Source: three-view drawing plus pictorial views. Frame: mm from the lowest corner of the part. A direction names the side the tool comes from. Coordinates: 2 decimals unless noted, no trailing zeros. Write each loop counter-clockwise with the first axis right and the second up, starting at its lowest first coordinate (ties: lowest second). Pieces come first, ordered by that corner, then holes. Notation, with made-up numbers: M 76.5,37 L 115.5,37 A24 cw 115.5,67 Z; hole C 26,3 d2. An arc over 180 degrees is marked long. Answer as a JSON object with one key per item and string values. Group by question number.
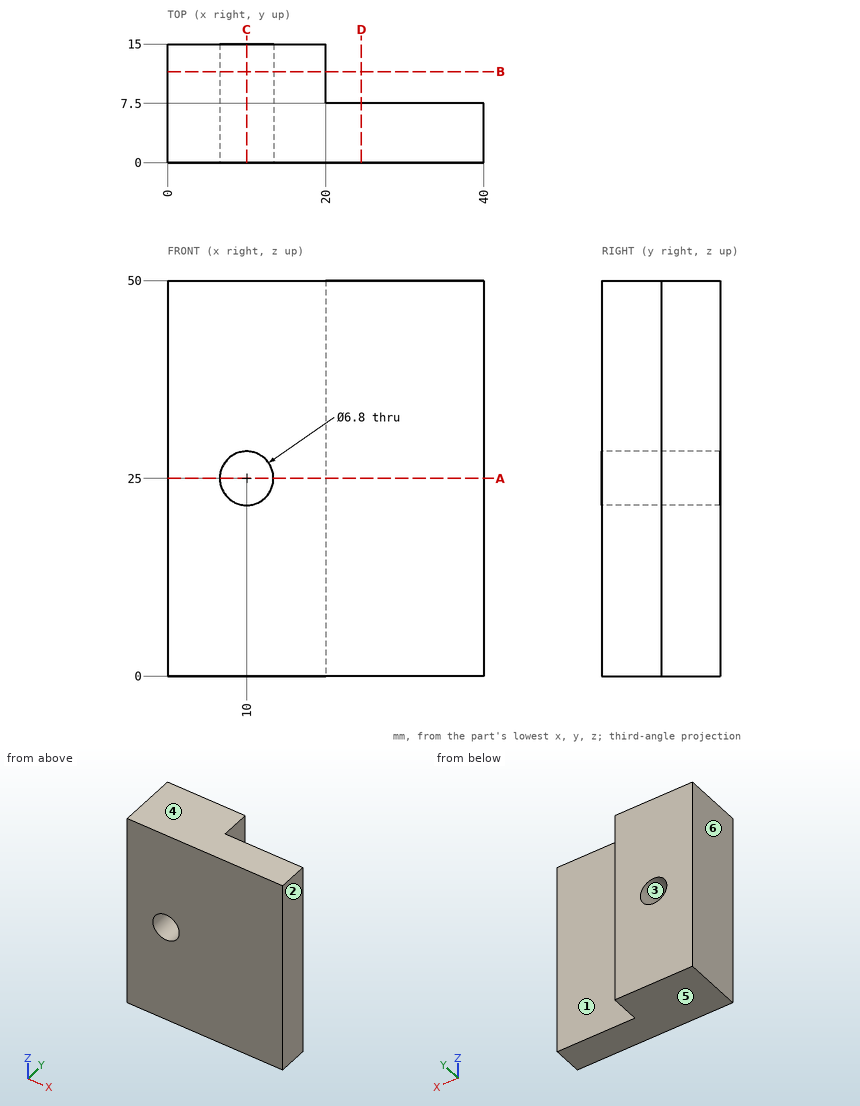
Q1. Pin query (flat end, axial travel): pin 1 Ø2 at (x, y) = (30.5, 2.5) entering from -Z; pin 2 Ø10 at (x, z) = (30, 34.5) entering from +Y. Return the tip coordinate at first contact, or that it passes through.
Q2. Section D-D, the plane x = 24.5. Return the cut outline in (y, z), and give its area (3 significant figures).
Q3. Draft query along Z for the marked faces 3, 4, 5 and 6. Return one class per face: released by +Z, released by -Z, zero draft, split by the parting line, or undercut.
Q4. Section B-B, the plane y = 11.5. Return the cut outline in (x, z).
Q5. Section A-A, the plane z = 25. Return the cut outline in (x, y), and give its area (3 significant figures).
Q6. Line query: line 1 (Z direction, x = 10, y = 7); line 2 (X direction, y = 6, z = 25); line 3 (Y direction, x = 22.5, z = 7). Output: solid intervals per line, ascending. Write a range as from..to.
Q7. Section C-C, the plane x = 10. Return the cut outline in (y, z), and give its area (3 significant figures).
Q8. Access query for the marked faces 1 and 2. Directions: +Z, -Z, +X, -X, +Y, -Y. A direction counts if a zero-diameter tool reaches every point of the face in a straight line with its end or side. Return the directions, or none.
Filled in:
{
 "1": {"pin 1": "z = 0", "pin 2": "y = 7.5"},
 "2": {"outline": "M 0,0 L 7.5,0 L 7.5,50 L 0,50 Z", "area": "375 mm^2"},
 "3": {"face 3": "undercut", "face 4": "released by +Z", "face 5": "released by -Z", "face 6": "zero draft"},
 "4": {"outline": "M 0,0 L 20,0 L 20,50 L 0,50 Z; hole C 10,25 d6.8"},
 "5": {"outline": "M 0,0 L 6.6,0 L 6.6,15 L 0,15 Z; M 13.4,0 L 40,0 L 40,7.5 L 20,7.5 L 20,15 L 13.4,15 Z", "area": "348 mm^2"},
 "6": {"line 1": "0..21.6, 28.4..50", "line 2": "0..6.6, 13.4..40", "line 3": "0..7.5"},
 "7": {"outline": "M 0,0 L 15,0 L 15,21.6 L 0,21.6 Z; M 0,28.4 L 15,28.4 L 15,50 L 0,50 Z", "area": "648 mm^2"},
 "8": {"face 1": "+Z, -Z, +X, +Y", "face 2": "+Z, -Z, +X, +Y, -Y"}
}
